```python
from build123d import *

# Parameters (mm, degrees)
F0_R        = 2.5
F1_DEPTH    = 2
F2_DEPTH    = 4
F3_T1_DEPTH = 2
F4_T1_DEPTH = 32.4048198529
F4_T3_DEPTH = 32.4048198529
F4_T5_DEPTH = 32.4048198529
F5_SIZE2    = 2.309391
F5_SIZE     = 3.99999
F5_2_SIZE2  = 2.309391
F5_2_SIZE   = 3.99999
F5_3_SIZE2  = 2.309391
F5_3_SIZE   = 3.99999
F6_SIZE     = 2.5
F7_SIZE     = 2


# Not quite as in the source:
# - a fillet or chamfer that OpenCascade refuses, or shapes differently, is made with other operations: its cross-section is extruded or revolved along the edge and cut away or added
# - a fillet or chamfer is up to 0.001 mm smaller than in the source, because OpenCascade refuses the exact size


with BuildPart() as f1:
    # F0 (on Top) → F1 (new body)
    with BuildSketch(Plane.XY):
        with BuildLine():
            ThreePointArc((-10.8535175815, -16.798843892), (-10, -17.3205080757), (-9.1214667739, -17.798843892))
            Line((-9.1214667739, -17.798843892), (-1.583464339, -4.7426406871))
            ThreePointArc((-1.583464339, -4.7426406871), (-2.5, -4.3301270189), (-3.3155151466, -3.7426406871))
            Line((-3.3155151466, -3.7426406871), (-10.8535175815, -16.798843892))
        make_face()
        with BuildLine():
            Line((-1.583464339, 4.7426406871), (-9.1214667739, 17.798843892))
            ThreePointArc((-9.1214667739, 17.798843892), (-10, 17.3205080757), (-10.8535175815, 16.798843892))
            Line((-10.8535175815, 16.798843892), (-3.3155151466, 3.7426406871))
            ThreePointArc((-3.3155151466, 3.7426406871), (-2.5, 4.3301270189), (-1.583464339, 4.7426406871))
        make_face()
        with BuildLine():
            ThreePointArc((20, 0), (19.9937451108, 0.5001564212), (19.9749843554, 1))
            Line((19.9749843554, 1), (4.8989794856, 1))
            ThreePointArc((4.8989794856, 1), (4.974680765, 0.50254481), (5, 0))
            ThreePointArc((5, 0), (4.974680765, -0.50254481), (4.8989794856, -1))
            Line((4.8989794856, -1), (19.9749843554, -1))
            ThreePointArc((19.9749843554, -1), (19.9937451108, -0.5001564212), (20, 0))
        make_face()
        with BuildLine():
            ThreePointArc((5, 0), (4.974680765, 0.50254481), (4.8989794856, 1))
            ThreePointArc((4.8989794856, 1), (2.5, 4.3301270189), (-1.583464339, 4.7426406871))
            ThreePointArc((-1.583464339, 4.7426406871), (-2.5, 4.3301270189), (-3.3155151466, 3.7426406871))
            ThreePointArc((-3.3155151466, 3.7426406871), (-5, 0), (-3.3155151466, -3.7426406871))
            ThreePointArc((-3.3155151466, -3.7426406871), (-2.5, -4.3301270189), (-1.583464339, -4.7426406871))
            ThreePointArc((-1.583464339, -4.7426406871), (2.5, -4.3301270189), (4.8989794856, -1))
            ThreePointArc((4.8989794856, -1), (4.974680765, -0.50254481), (5, 0))
        make_face()
        Circle(F0_R, mode=Mode.SUBTRACT)
    extrude(amount=F1_DEPTH)

    # F0 (on Top) → F2 (join)
    with BuildSketch(Plane.XY):
        with BuildLine():
            Line((0, 20), (0, 30))
            ThreePointArc((0, 30), (-15, 25.9807621135), (-25.9807621135, 15))
            Line((-25.9807621135, 15), (-17.3205080757, 10))
            ThreePointArc((-17.3205080757, 10), (-14.4913767462, 13.7840487521), (-10.8535175815, 16.798843892))
            ThreePointArc((-10.8535175815, 16.798843892), (-10, 17.3205080757), (-9.1214667739, 17.798843892))
            ThreePointArc((-9.1214667739, 17.798843892), (-4.6916480132, 19.4419247741), (0, 20))
        make_face()
        with BuildLine():
            ThreePointArc((25.9807621135, -15), (28.9777747887, -7.7645713531), (30, 0))
            ThreePointArc((30, 0), (28.9777747887, 7.7645713531), (25.9807621135, 15))
            Line((25.9807621135, 15), (17.3205080757, 10))
            ThreePointArc((17.3205080757, 10), (19.1830247594, 5.657876022), (19.9749843554, 1))
            ThreePointArc((19.9749843554, 1), (19.9937451108, 0.5001564212), (20, 0))
            ThreePointArc((20, 0), (19.9937451108, -0.5001564212), (19.9749843554, -1))
            ThreePointArc((19.9749843554, -1), (19.1830247594, -5.657876022), (17.3205080757, -10))
            Line((17.3205080757, -10), (25.9807621135, -15))
        make_face()
        with BuildLine():
            ThreePointArc((-25.9807621135, -15), (-15, -25.9807621135), (0, -30))
            Line((0, -30), (0, -20))
            ThreePointArc((0, -20), (-4.6916480132, -19.4419247741), (-9.1214667739, -17.798843892))
            ThreePointArc((-9.1214667739, -17.798843892), (-10, -17.3205080757), (-10.8535175815, -16.798843892))
            ThreePointArc((-10.8535175815, -16.798843892), (-14.4913767462, -13.7840487521), (-17.3205080757, -10))
            Line((-17.3205080757, -10), (-25.9807621135, -15))
        make_face()
    extrude(amount=F2_DEPTH)

    # F3: fillet of radius 5 on 12 edges, made by hand

    # F3_s2 → F3_t1 (join)
    with BuildSketch(Plane.XY):
        with BuildLine():
            ThreePointArc((-2.2369481596, 19.8745078664), (-6.1410694312, 17.1594186926), (-6.0078381387, 12.4058808998))
            Line((-6.0078381387, 12.4058808998), (-9.1214667739, 17.798843892))
            ThreePointArc((-9.1214667739, 17.798843892), (-5.7732566792, 19.148616329), (-2.2369481596, 19.8745078664))
        make_face()
        with BuildLine():
            ThreePointArc((-16.0933546202, 11.8745078664), (-11.7899577863, 13.8980314801), (-7.7398889462, 11.4058808998))
            Line((-7.7398889462, 11.4058808998), (-10.8535175815, 16.798843892))
            ThreePointArc((-10.8535175815, 16.798843892), (-13.6965598486, 14.5740951113), (-16.0933546202, 11.8745078664))
        make_face()
        with BuildLine():
            ThreePointArc((18.3303027798, 8), (17.9310272175, 3.2613872125), (13.7477270849, 1))
            Line((13.7477270849, 1), (19.9749843554, 1))
            ThreePointArc((19.9749843554, 1), (19.4698165279, 4.5745212177), (18.3303027798, 8))
        make_face()
        with BuildLine():
            ThreePointArc((13.7477270849, -1), (17.9310272175, -3.2613872125), (18.3303027798, -8))
            ThreePointArc((18.3303027798, -8), (19.4698165279, -4.5745212177), (19.9749843554, -1))
            Line((19.9749843554, -1), (13.7477270849, -1))
        make_face()
        with BuildLine():
            ThreePointArc((-16.0933546202, -11.8745078664), (-11.7899577863, -13.8980314801), (-7.7398889462, -11.4058808998))
            Line((-7.7398889462, -11.4058808998), (-10.8535175815, -16.798843892))
            ThreePointArc((-10.8535175815, -16.798843892), (-13.6965598486, -14.5740951113), (-16.0933546202, -11.8745078664))
        make_face()
        with BuildLine():
            ThreePointArc((-2.2369481596, -19.8745078664), (-6.1410694312, -17.1594186926), (-6.0078381387, -12.4058808998))
            Line((-6.0078381387, -12.4058808998), (-9.1214667739, -17.798843892))
            ThreePointArc((-9.1214667739, -17.798843892), (-5.7732566792, -19.148616329), (-2.2369481596, -19.8745078664))
        make_face()
        with BuildLine():
            ThreePointArc((-3.1339745962, 7.4282032303), (-1.5587969348, 5.7556435797), (0.5980762114, 4.9641016151))
            ThreePointArc((0.5980762114, 4.9641016151), (-0.5049838375, 4.9744337692), (-1.583464339, 4.7426406871))
            Line((-1.583464339, 4.7426406871), (-3.1339745962, 7.4282032303))
        make_face()
        with BuildLine():
            ThreePointArc((8, 1), (5.7639320225, 1.527864045), (4, 3))
            ThreePointArc((4, 3), (4.5604779323, 2.0498880528), (4.8989794856, 1))
            Line((4.8989794856, 1), (8, 1))
        make_face()
        with BuildLine():
            ThreePointArc((-4.8660254038, 6.4282032303), (-4.2051350877, 4.2277795347), (-4.5980762114, 1.9641016151))
            ThreePointArc((-4.5980762114, 1.9641016151), (-4.0554940948, 2.9245457164), (-3.3155151466, 3.7426406871))
            Line((-3.3155151466, 3.7426406871), (-4.8660254038, 6.4282032303))
        make_face()
        with BuildLine():
            ThreePointArc((-4.5980762114, -1.9641016151), (-4.2051350877, -4.2277795347), (-4.8660254038, -6.4282032303))
            Line((-4.8660254038, -6.4282032303), (-3.3155151466, -3.7426406871))
            ThreePointArc((-3.3155151466, -3.7426406871), (-4.0554940948, -2.9245457164), (-4.5980762114, -1.9641016151))
        make_face()
        with BuildLine():
            ThreePointArc((-3.1339745962, -7.4282032303), (-1.5587969348, -5.7556435797), (0.5980762114, -4.9641016151))
            ThreePointArc((0.5980762114, -4.9641016151), (-0.5049838375, -4.9744337692), (-1.583464339, -4.7426406871))
            Line((-1.583464339, -4.7426406871), (-3.1339745962, -7.4282032303))
        make_face()
        with BuildLine():
            ThreePointArc((4, -3), (5.7639320225, -1.527864045), (8, -1))
            Line((8, -1), (4.8989794856, -1))
            ThreePointArc((4.8989794856, -1), (4.5604779323, -2.0498880528), (4, -3))
        make_face()
    extrude(amount=F3_T1_DEPTH)

    # F4: chamfer of 2.5 x 4.3301270189 on 3 edges, made by hand

    # F4_s2 → F4_t1 (cut)
    with BuildSketch(Plane(origin=(-7.6189364958, -4.3987950368, 0), x_dir=(0, 0, 1), z_dir=(-0.8660254038, -0.5, 0))):
        Polygon((-0.3301270189, 0), (4, -2.5), (4, 0), align=None)
    extrude(amount=F4_T1_DEPTH, mode=Mode.SUBTRACT)

    # F4_s4 → F4_t3 (cut)
    with BuildSketch(Plane.XZ.offset(-41.2024099265)):
        Polygon((-2.5, 4), (0, -0.3301270189), (0, 4), align=None)
    extrude(amount=F4_T3_DEPTH, mode=Mode.SUBTRACT)

    # F4_s6 → F4_t5 (cut)
    with BuildSketch(Plane(origin=(7.6189364958, -4.3987950368, 0), x_dir=(0, 0, 1), z_dir=(0.8660254038, -0.5, 0))):
        Polygon((-0.3301270189, 0), (4, -2.5), (4, 0), align=None)
    extrude(amount=F4_T5_DEPTH, mode=Mode.SUBTRACT)

    # F5 (size 4 and 2.3094010768 in the source; OpenCascade refuses exactly that, so slightly less here)
    f5_edges = [f1.edges().sort_by_distance(p)[0] for p in [
        (21.650635, 12.5, 4),
    ]]
    f5_side = f1.faces().sort_by_distance((21.650635, 12.5, 2))[0]
    chamfer(f5_edges, length=F5_SIZE, length2=F5_SIZE2, reference=f5_side)

    # F5#2 (size 4 and 2.3094010768 in the source; OpenCascade refuses exactly that, so slightly less here)
    f5_2_edges = [f1.edges().sort_by_distance(p)[0] for p in [
        (-21.650635, 12.5, 4),
    ]]
    f5_2_side = f1.faces().sort_by_distance((-21.650635, 12.5, 2))[0]
    chamfer(f5_2_edges, length=F5_2_SIZE, length2=F5_2_SIZE2, reference=f5_2_side)

    # F5#3 (size 4 and 2.3094010768 in the source; OpenCascade refuses exactly that, so slightly less here)
    f5_3_edges = [f1.edges().sort_by_distance(p)[0] for p in [
        (0, -25, 4),
    ]]
    f5_3_side = f1.faces().sort_by_distance((0, -25, 2))[0]
    chamfer(f5_3_edges, length=F5_3_SIZE, length2=F5_3_SIZE2, reference=f5_3_side)

    # F6
    f6_edges = [f1.edges().sort_by_distance(p)[0] for p in [
        (-20.399464, 14.444291, 4),
        (-2.5, 24.869393, 4),
        (22.708855, 10.444309, 4),
        (22.787526, -10.269633, 4),
        (-2.309391, -24.8886, 4),
        (-20.287526, -14.59976, 4),
    ]]
    chamfer(f6_edges, length=F6_SIZE)

    # F7
    f7_edges = [f1.edges().sort_by_distance(p)[0] for p in [
        (-5, 24.472658, 4),
        (-18.823804, 16.421335, 4),
        (23.633195, 8.091225, 4),
        (23.693943, -7.906202, 4),
        (-4.809391, -24.51256, 4),
        (-18.693943, -16.566456, 4),
    ]]
    chamfer(f7_edges, length=F7_SIZE)


solid = f1.part
```
Verification items for the finished model (mm, model axes). A direction names the side the tool comes from. Round coordinates to 2 decimals unless told otherwise and drop trailing zeros. Write each loop counter-clockwise with the first axis right and the second up, starting at its lowest first coordinate (ties: lowest second). Pieces come first, ordered by that corner, then holes. Notation, with made-up numbers: (-14, -21) - (27, -21) arc R16 cw to (27, -2) - close; hole circle Ø10 at (9, -36.75). An arc over 180 degrees is marked (long way). Answer as a JSON object with one key per item and string values. Group by question number.
Q1. Tool access check on faces 1 (the flat face through (1, -3, 2)), 2 (the flat face through (22.597, -10.422, 2.426)), 3 (the flat face through (-2.273, 24.924, 2.426)), 4 (the cylindrical face through (-11.86, -13.9, 0.99)). Record the directions out of +Z, -Z, +X, -X, +Y, -Y that give a thin tool (end or side, any length) a straight path to the whole face; none if there is none.
Q2. Section check B-B, the plane x = 13. Enter the section's corners in (y, z), plus the area to 3 significant figures.
Q3. Thickness scan on line 1 (Z direction, x = -1.5, y = 23); line 2 (Y direction, x = -14, z = 2.9); line 3 (Y direction, x = 0, z = 1.05). Record the ranges inside material, lowest first.
Q4. Go/stop test with flat-tipped pins: pin 1 Ø1.5 at (x, z) = (20, 1.5) entering from +Y; pin 2 Ø1 at (x, z) = (12, 0.5) entering from +Y; pin 3 Ø11 at (x, y) = (-6, 6) entering from +Z. Record where each tip stops, or that it passes through.
Q5. Mould release check, pull along X, two halves, no side actions. Record for faces 5 (the flat face through (11, 1, 1)), 6 (the flat face through (23.538, -7.632, 3.507)), 7 (the flat face through (-2.082, -24.943, 2.426)): released by +X, released by -X, zero draft, split by the parting line, or undercut.
Found:
{
 "1": {"face 1": "+Z", "face 2": "+Z, -Y", "face 3": "+Z, +X, +Y", "face 4": "+Z, -Z"},
 "2": {"outline": "(-1, 0) - (1, 0) - (1, 2) - (-1, 2) - close", "area": "4.00 mm^2"},
 "3": {"line 1": "z = 0 to 1.98", "line 2": "y = -26.53 to -14.28, 14.28 to 26.53", "line 3": "y = -5.07 to -2.5, 2.5 to 5.07"},
 "4": {"pin 1": "stops at y = 11.21", "pin 2": "stops at y = 1", "pin 3": "stops at z = 2"},
 "5": {"face 5": "undercut", "face 6": "released by -X", "face 7": "released by +X"}
}
